Model file for the job. Use its own axes, mm. Face numbers are marked on the shaded views. A direction names the side the tool comes from. Coordinates: 2 decimals unless noted, no trailing zeros. Loops run counter-clockwise (first coordinate to the right, second up) from the corner with the lowest first, then second, coordinate; pieces in that order, holes last.
from build123d import *

# Parameters (mm, degrees)
SKETCH1_W          = 6.95
SKETCH1_H          = 0.5
SKETCH1_W_2        = 2.8
SKETCH1_H_2        = 1.2
CUT_EXTRUDE2_START = 2
CUT_EXTRUDE2_DEPTH = 2
SKETCH3_W          = 1.17
SKETCH3_H          = 1.465
SKETCH3_H_2        = 1.17
SKETCH3_W_2        = 1.465
CUT_EXTRUDE3_DEPTH = 4.3
FILLET1_R          = 0.3
FILLET2_R          = 1
FILLET3_R          = 2


with BuildPart() as part:
    # Sketch1 → Revolve1 (revolve)
    with BuildSketch(Plane(origin=(0, 0, 0), x_dir=(1, 0, 0), z_dir=(0, 1, 0)), mode=Mode.PRIVATE) as revolve1_sk:
        with BuildLine():
            Line((2.8, 0), (0, 0))
            Line((0, 0), (0, -4.5))
            ThreePointArc((0, -4.5), (4.631751828, -4.625091174), (9.25, -5))
            Line((9.25, -5), (11.25, -5))
            Line((11.25, -5), (11.25, 0))
            Line((11.25, 0), (9.75, 0))
            Line((9.75, 0), (9.75, -3.1))
            Line((9.75, -3.1), (9.75, -3.6))
            Line((9.75, -3.6), (2.8, -3.6))
            Line((2.8, -3.6), (2.8, -3.1))
            Line((2.8, -3.1), (2.8, 0))
        make_face()
        with Locations((6.275, -3.35)):
            Rectangle(SKETCH1_W, SKETCH1_H)
        with Locations((1.4, 0.6)):
            Rectangle(SKETCH1_W_2, SKETCH1_H_2)
    revolve(revolve1_sk.sketch.rotate(Axis((0, 0, 0), (0, 0, 1)), 180), axis=Axis((0, 0, 0), (0, 0, 1)))

    # Sketch2 → Cut-Extrude2 (cut)
    with BuildSketch(Plane.XY.offset(CUT_EXTRUDE2_START)):
        with BuildLine():
            Line((8.558921926, 7.350980651), (7.350980651, 8.558921926))
            Line((7.350980651, 8.558921926), (4.669834629, 8.558921926))
            ThreePointArc((4.669834629, 8.558921926), (6.894291117, 6.894291117), (8.558921926, 4.669834629))
            Line((8.558921926, 4.669834629), (8.558921926, 7.350980651))
        make_face()
        Polygon((7.350980651, 8.558921926), (6.01040764, 9.899494937), (4.669834629, 8.558921926), align=None)
        Polygon((9.899494937, 6.01040764), (8.558921926, 7.350980651), (8.558921926, 4.669834629), align=None)
        Polygon((9.899494937, -6.01040764), (8.558921926, -4.669834629), (8.558921926, -7.350980651), align=None)
        with BuildLine():
            Line((8.558921926, -7.350980651), (8.558921926, -4.669834629))
            ThreePointArc((8.558921926, -4.669834629), (6.894291117, -6.894291117), (4.669834629, -8.558921926))
            Line((4.669834629, -8.558921926), (7.350980651, -8.558921926))
            Line((7.350980651, -8.558921926), (8.558921926, -7.350980651))
        make_face()
        Polygon((7.350980651, -8.558921926), (4.669834629, -8.558921926), (6.01040764, -9.899494937), align=None)
        Polygon((-6.01040764, -9.899494937), (-4.669834629, -8.558921926), (-7.350980651, -8.558921926), align=None)
        with BuildLine():
            ThreePointArc((-4.669834629, -8.558921926), (-6.894291117, -6.894291117), (-8.558921926, -4.669834629))
            Line((-8.558921926, -4.669834629), (-8.558921926, -7.350980651))
            Line((-8.558921926, -7.350980651), (-7.350980651, -8.558921926))
            Line((-7.350980651, -8.558921926), (-4.669834629, -8.558921926))
        make_face()
        Polygon((-8.558921926, -7.350980651), (-8.558921926, -4.669834629), (-9.899494937, -6.01040764), align=None)
        Polygon((-9.899494937, 6.01040764), (-8.558921926, 4.669834629), (-8.558921926, 7.350980651), align=None)
        with BuildLine():
            ThreePointArc((-8.558921926, 4.669834629), (-6.894291117, 6.894291117), (-4.669834629, 8.558921926))
            Line((-4.669834629, 8.558921926), (-7.350980651, 8.558921926))
            Line((-7.350980651, 8.558921926), (-8.558921926, 7.350980651))
            Line((-8.558921926, 7.350980651), (-8.558921926, 4.669834629))
        make_face()
        Polygon((-7.350980651, 8.558921926), (-4.669834629, 8.558921926), (-6.01040764, 9.899494937), align=None)
    extrude(amount=-CUT_EXTRUDE2_DEPTH, mode=Mode.SUBTRACT)

    # Sketch3 → Cut-Extrude3 (cut)
    with BuildSketch(Plane(origin=(0, 0, -1.2), x_dir=(-1, 0, 0), z_dir=(0, 0, -1))):
        with Locations((0, 1.3175)):
            Rectangle(SKETCH3_W, SKETCH3_H)
        Rectangle(SKETCH3_W, SKETCH3_H_2)
        with Locations((0, -1.3175)):
            Rectangle(SKETCH3_W, SKETCH3_H)
        with Locations((-1.3175, 0)):
            Rectangle(SKETCH3_W_2, SKETCH3_H_2)
        with Locations((1.3175, 0)):
            Rectangle(SKETCH3_W_2, SKETCH3_H_2)
    extrude(amount=-CUT_EXTRUDE3_DEPTH, mode=Mode.SUBTRACT)

    # Fillet1
    fillet1_edges = [part.edges().sort_by_distance(p)[0] for p in [
        (0.585, 0.585, 0.95),
        (0.585, -0.585, 0.95),
        (-0.585, -0.585, 0.95),
        (-0.585, 0.585, 0.95),
    ]]
    fillet(fillet1_edges, radius=FILLET1_R)

    # Fillet2
    fillet2_edges = [part.edges().sort_by_distance(p)[0] for p in [
        (9.75, 0, 3.1),
    ]]
    fillet(fillet2_edges, radius=FILLET2_R)

    # Fillet3
    fillet3_edges = [part.edges().sort_by_distance(p)[0] for p in [
        (11.25, 0, 5),
    ]]
    fillet(fillet3_edges, radius=FILLET3_R - 0.0001)  # a hair under: the kernel refuses the full size


solid = part.part
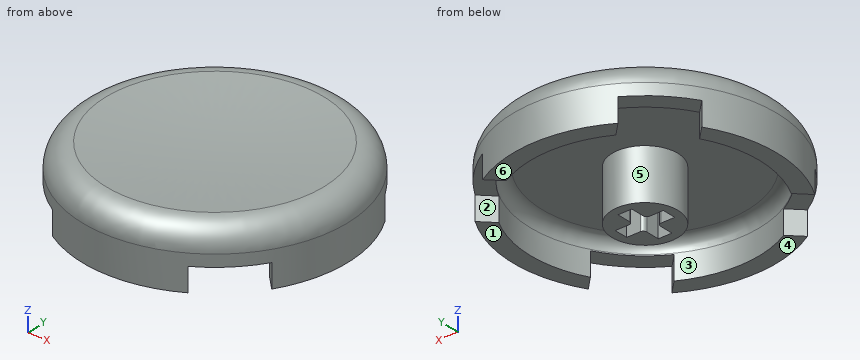
Q1. Mould opens along Y. For the marked faces 1, 2 and 3 say: +Y half, -Y half, draft (parallel to the pull), parting line (faces both ways), or undercut.
Answers:
face 1: draft
face 2: +Y half
face 3: undercut
Q2. Which spindle directions (+Z, -Z, +X, -X, +Y, -Y) get a long thin tool onto all of the face, cutting with end or side? Do the marked faces 4, 5 and 6. Say none if no direction does.
Answers:
face 4: -Z, +X, -X, -Y
face 5: -Z
face 6: -Z, +X, -X, +Y
Q3. Slice it at B-B (z = 2.5). List the corners of the cut face in (x, y) (3 decimals).
Answers:
outline: circle Ø22.5 at (0, 0); circle Ø5.6 at (0, 0); hole circle Ø19.333 at (0, 0); hole (-2.05, -0.585) - (-0.885, -0.585) arc R0.3 cw to (-0.585, -0.885) - (-0.585, -2.05) - (0.585, -2.05) - (0.585, -0.885) arc R0.3 cw to (0.885, -0.585) - (2.05, -0.585) - (2.05, 0.585) - (0.885, 0.585) arc R0.3 cw to (0.585, 0.885) - (0.585, 2.05) - (-0.585, 2.05) - (-0.585, 0.885) arc R0.3 cw to (-0.885, 0.585) - (-2.05, 0.585) - close
Q4. Slice it at D-D (z = 3.75). List the corners of the cut face in (x, y).
Answers:
outline: circle Ø22.21 at (0, 0)
Q5. Flat gauge pins, fed straight in: P1, Ø1.3, axis at x = 1.5, z = 1.5, coming from the +Y side; P2, Ø1.3, axis at x = 9.5, y = -2, coming from the -Z side; P3, Ø1.5, axis at x = 7, y = -4, coming from the +Z side. Where does each tip first touch, or does it go through?
Answers:
P1: stops at y = 11.22
P2: stops at z = 0
P3: stops at z = 4.95
Q6. Drill centre lines: line 1 (Y direction, x = 0, z = 1.3); line 2 (Y direction, x = -0.75, z = 1.5); line 3 (Z direction, x = 3.75, y = 3.75). Where is each one in solid material? Low to high.
Answers:
line 1: y = -11.25 to -9.75, -2.8 to -2.05, 2.05 to 2.8, 9.75 to 11.25
line 2: y = -11.22 to -9.72, -2.7 to -0.62, 0.62 to 2.7, 9.72 to 11.22
line 3: z = 3.1 to 4.66
